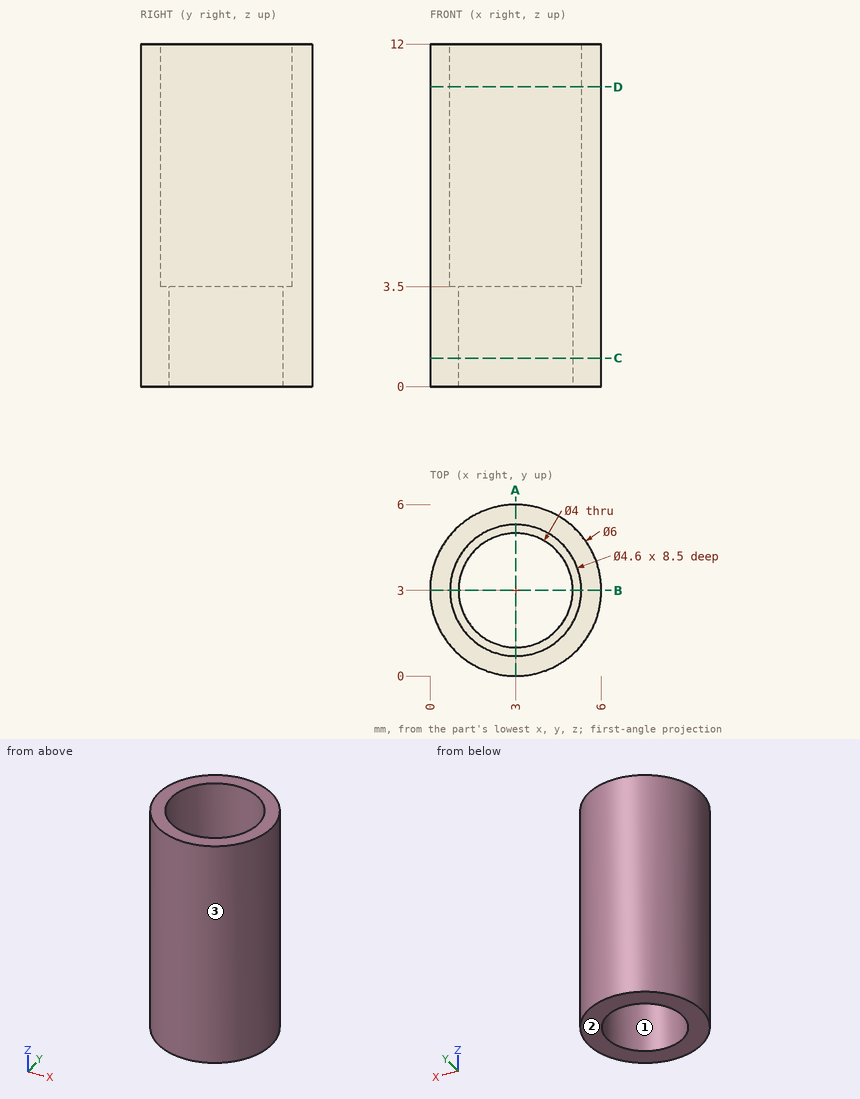
The drawing under review shows one solid part. Ordinate dimensions are in mm from its lowest x, y, z. Coordinates: 2 decimals unless noted, no trailing zeros. Write each loop counter-clockwise with the first axis right and the second up, starting at its lowest first coordinate (ties: lowest second). Pieces come first, ordered by that corner, then holes. Notation, with made-up numbers: M -8.75,-3 L -0.75,-3 A25 cw -0.75,15 Z; hole C 48.25,1.25 d3. An arc over 180 degrees is marked long. Answer as a JSON object with one key per item and string values.
Item 1: Draft analysis for pull direction Y (two halves, no side actions). For the marked faces 1, 2 and 3, state which applies: pulls with the +Y half, pulls with the -Y half, needs draft (parallel to the pull), parting line crosses it, or undercut.
Outcome:
{"face 1": "undercut", "face 2": "needs draft", "face 3": "parting line crosses it"}
Item 2: Add section C-C, the plane z = 1. Give the boundary of the cut face in (x, y).
Outcome:
{"outline": "C 3,3 d6; hole C 3,3 d4"}
Item 3: Add section A-A, the plane x = 3. Give the boundary of the cut face in (y, z), and give its area (3 significant figures).
Outcome:
{"outline": "M 0,0 L 1,0 L 1,3.5 L 0.7,3.5 L 0.7,12 L 0,12 Z; M 5,0 L 6,0 L 6,12 L 5.3,12 L 5.3,3.5 L 5,3.5 Z", "area": "18.9 mm²"}
Item 4: Insertion check: pin 1 Ø3 at (x, z) = (5, 1.5) entering from -Y; pin 2 Ø1.5 at (x, y) = (4.5, 2.5) entering from +Z; pin 3 Ø3.5 at (x, y) = (3, 2.5) entering from +Z. Each pin has a flat end and moves straight along its axis. Give the tip position at first contact, or say it passes through.
Outcome:
{"pin 1": "y = 0.04", "pin 2": "z = 12", "pin 3": "z = 3.5"}
Item 5: Add section D-D, the plane z = 10.5. Give the boundary of the cut face in (x, y), and give its area (3 significant figures).
Outcome:
{"outline": "C 3,3 d6; hole C 3,3 d4.6", "area": "11.7 mm²"}
Item 6: Wall thickness on probe 1 along Y at (x, z) = (3, 2.1); probe 2 along X at (y, z) = (4.7, 3); probe 3 along X at (y, z) = (2, 7.5): over which ranges is each line inside the solid? List them lowest first.
Outcome:
{"probe 1": "0 to 1, 5 to 6", "probe 2": "0.53 to 1.95, 4.05 to 5.47", "probe 3": "0.17 to 0.93, 5.07 to 5.83"}
